Can you work these out from the model? Positions are in its coordinate system, mm. Round coordinates to 2 decimals unless told otherwise and drop trailing zeros. Loops run counter-clockwise (first coordinate to the right, second up) from the corner with the lowest first, then second, coordinate; pieces in that order, holes last.
```python
from build123d import *

# Parameters (mm, degrees)
F0_R     = 1.5
F1_DEPTH = 4
F3_DEPTH = 25
F4_W     = 4
F4_H     = 10
F5_DEPTH = 4


with BuildPart() as f1:
    # F0 (on Top) → F1 (new body)
    with BuildSketch(Plane.XY):
        with BuildLine():
            ThreePointArc((-25.5, -18), (-25.93934, -16.93934), (-27, -16.5))
            ThreePointArc((-27, -16.5), (-28.06066, -19.06066), (-25.5, -18))
        make_face()
        with BuildLine():
            Line((-45, 0), (-55.5, 0))
            ThreePointArc((-55.5, 0), (-45, -10.5), (-34.5, 0))
            Line((-34.5, 0), (-45, 0))
        make_face()
        Polygon((-75, -30), (75, -30), (75, 30), (-75, 30), (-75, 0), align=None)
        with Locations((-63, -18)):
            Circle(F0_R, mode=Mode.SUBTRACT)
        with BuildLine():
            ThreePointArc((-25.5, -18), (-28.06066, -19.06066), (-27, -16.5))
            ThreePointArc((-27, -16.5), (-25.93934, -16.93934), (-25.5, -18))
        make_face(mode=Mode.SUBTRACT)
        with BuildLine():
            ThreePointArc((-34.5, 0), (-45, -10.5), (-55.5, 0))
            ThreePointArc((-55.5, 0), (-45, 10.5), (-34.5, 0))
        make_face(mode=Mode.SUBTRACT)
        with Locations((-63, 18)):
            Circle(F0_R, mode=Mode.SUBTRACT)
        with Locations((-27, 18)):
            Circle(F0_R, mode=Mode.SUBTRACT)
    extrude(amount=F1_DEPTH)

    # F2 (on face) → F3 (cut)
    with BuildSketch(Plane(origin=(0, 0, 0), x_dir=(1, 0, 0), z_dir=(0, 0, -1))):
        with BuildLine():
            ThreePointArc((55, -1.5), (57.291288, -1.114378), (59.330127, 0))
            Line((59.330127, 0), (55, 0))
            Line((55, 0), (55, -1.5))
        make_face()
        with BuildLine():
            ThreePointArc((62, -15.5), (59.949747, -10.550253), (55, -8.5))
            ThreePointArc((55, -8.5), (50.050253, -20.449747), (62, -15.5))
        make_face()
        with BuildLine():
            ThreePointArc((12, -10.5), (9.949747, -5.550253), (5, -3.5))
            ThreePointArc((5, -3.5), (0.050253, -15.449747), (12, -10.5))
        make_face()
        with BuildLine():
            ThreePointArc((12, 10.5), (0.050253, 15.449747), (5, 3.5))
            ThreePointArc((5, 3.5), (9.949747, 5.550253), (12, 10.5))
        make_face()
        with BuildLine():
            ThreePointArc((37, 15.5), (25.050253, 20.449747), (30, 8.5))
            ThreePointArc((30, 8.5), (34.949747, 10.550253), (37, 15.5))
        make_face()
        with BuildLine():
            ThreePointArc((37, -3.5), (36.761481, -1.688267), (36.062178, 0))
            Line((36.062178, 0), (30, 0))
            Line((30, 0), (23.937822, 0))
            ThreePointArc((23.937822, 0), (28.188267, -10.261481), (37, -3.5))
        make_face()
        with BuildLine():
            Line((30, 0), (36.062178, 0))
            ThreePointArc((36.062178, 0), (33.5, 2.562178), (30, 3.5))
            Line((30, 3.5), (30, 0))
        make_face()
        with BuildLine():
            Line((55, 0), (59.330127, 0))
            ThreePointArc((59.330127, 0), (61.297257, 2.443113), (62, 5.5))
            ThreePointArc((62, 5.5), (51.943113, 11.797257), (50.669873, 0))
            Line((50.669873, 0), (55, 0))
        make_face()
        with BuildLine():
            Line((55, -1.5), (55, 0))
            Line((55, 0), (50.669873, 0))
            ThreePointArc((50.669873, 0), (52.708712, -1.114378), (55, -1.5))
        make_face()
        with BuildLine():
            Line((23.937822, 0), (30, 0))
            Line((30, 0), (30, 3.5))
            ThreePointArc((30, 3.5), (26.5, 2.562178), (23.937822, 0))
        make_face()
    extrude(amount=-F3_DEPTH, mode=Mode.SUBTRACT)

    # F4 (on face) → F5 (join)
    with BuildSketch(Plane(origin=(0, 0, 0), x_dir=(1, 0, 0), z_dir=(0, 0, -1))):
        Polygon((-75, -5), (-75, 0), (-75, 5), (-79, 5), (-79, -5), align=None)
        Polygon((-75, 20), (-75, 25), (-79, 25), (-79, 15), (-75, 15), align=None)
        Polygon((-75, -15), (-79, -15), (-79, -25), (-75, -25), (-75, -20), align=None)
        with Locations((77, 0)):
            Rectangle(F4_W, F4_H)
        with Locations((77, -20)):
            Rectangle(F4_W, F4_H)
        with Locations((77, 20)):
            Rectangle(F4_W, F4_H)
        Polygon((-75, 33), (-75, 30), (0, 30), (75, 30), (75, 33), align=None)
    extrude(amount=-F5_DEPTH)


solid = f1.part
```
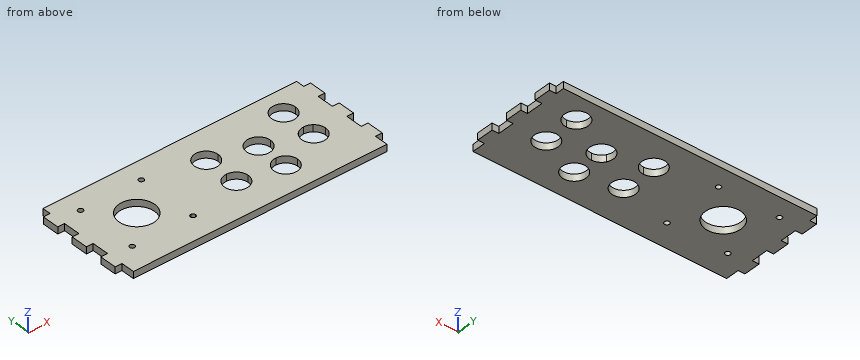
(1) Suppose I cut it at B-B (x = -63). Write out the boundary of the cut face in (y, z), then the cut area to 3 significant figures.
(2) Suppose I cut it at A-A (y = 21). Write out the boundary of the cut face in (x, z).
(3) For pin 1 (2 mm diameter, centred on y = -10, z = 0.5, fed in from +X); pin 2 (11 mm diameter, centred on x = 5, y = 10.5, fed in from +Z); pin 3 (2 mm diameter, centred on x = -77.5, z = 2, fed in from -Y); pin 4 (1.2 mm diameter, centred on x = -78, z = 2.5, fed in from +Y), each with a flat end and sliding along its axis, tell me the tip position at first contact or that it passes through.
(4) If I drill on line 1 (Y direction, x = 5, z = 1.3); line 2 (Y direction, x = 55, z = 1.5); line 3 (X direction, y = -15.5, z = 1.6), over which ranges is the centre line in solid material (lowest first)?
(5) Suppose I cut it at C-C (z = 2.55). Give the number of separate pieces and of enclosed holes in the cut face, then the cut area to 3 significant figures.
Check result:
1. outline: (-33, 0) - (-19.5, 0) - (-19.5, 4) - (-33, 4) - close; (-16.5, 0) - (16.5, 0) - (16.5, 4) - (-16.5, 4) - close; (19.5, 0) - (30, 0) - (30, 4) - (19.5, 4) - close
1. area: 228 mm2
2. outline: (-79, 0) - (50.67, 0) - (50.67, 4) - (-79, 4) - close; (59.33, 0) - (79, 0) - (79, 4) - (59.33, 4) - close
3. pin 1: stops at x = 75
3. pin 2: passes through
3. pin 3: stops at y = -25
3. pin 4: stops at y = 25
4. line 1: y = -33 to -17.5, -3.5 to 3.5, 17.5 to 30
4. line 2: y = -33 to -12.5, 1.5 to 8.5, 22.5 to 30
4. line 3: x = -79 to 0.1, 9.9 to 23, 37 to 79
5. separate pieces: 1
5. enclosed holes: 11
5. area: 8,390 mm2
